Autodesk Inventor part; units mm, degrees
ref_plane "YZ Plane" through (0, 0, 0) normal (1, 0, 0) x (0, 1, 0)
ref_plane "XZ Plane" through (0, 0, 0) normal (0, 1, 0) x (-1, 0, 0)
ref_plane "XY Plane" through (0, 0, 0) normal (0, 0, 1) x (1, 0, 0)
sketch "Sketch1" plane through (0, 0, 0) normal (0, 1, 0) x (-1, 0, 0)
  line L0 (0, 0) -> (0, -125.2474)
  line L1 (0, -125.2474) -> (-3.4036, -125.2474)
  line L2 (0, 0) -> (-3.4036, 0)
  line L3 (-3.4036, 0) -> (-6.5786, -31.3753)
  line L4 (-6.5786, -31.3753) -> (-1.778, -62.7507)
  line L5 (-1.778, -62.7507) -> (-6.5786, -93.8721)
  line L6 (-6.5786, -93.8721) -> (-3.4036, -125.2474)
  dimension "d0" = 125.2474
  dimension "d1" = 3.4036
  dimension "d2" = 3.4036
  dimension "d3" = 31.3754
  dimension "d4" = 62.7507
  dimension "d5" = 31.3754
  dimension "d6" = 3.175
  dimension "d7" = 3.175
extrude "Extrusion1" add sketch "Sketch1" along normal blind 7.3025
sketch "Sketch2" plane through (0, 0, 0) normal (0, 0, 1) x (1, 0, 0)
  line L0 (0, 0) -> (0, 7.3025)
  line L1 (3.4036, 0) -> (0, 0)
  line L2 (0, 7.3025) -> (1.651, 7.3025)
  line L3 (1.651, 7.3025) -> (1.651, 0)
  line L4 (1.651, 0) -> (0, 0)
  line L5 (0, 0) -> (0, 7.3025)
  dimension "d10" = 1.651
sketch "Sketch3" plane through (3.4036, 0, -125.2474) normal (0, 0, -1) x (-1, 0, 0)
  line L0 (0, 0) -> (3.4036, 0)
  line L1 (3.4036, 7.3025) -> (1.7526, 7.3025)
  line L2 (1.7526, 7.3025) -> (1.7526, 0)
  line L3 (1.7526, 0) -> (3.4036, 0)
  line L4 (3.4036, 0) -> (3.4036, 7.3025)
  dimension "d11" = 1.651
extrude "Extrusion2" add sketch "Sketch2" along normal blind 2.5654
extrude "Extrusion3" add sketch "Sketch3" along normal blind 2.5654
properties part number "long_insert_CPY1"
Could you check a few things on this model? Use its own coordinates, in mm. A direction names the side the tool comes from. Round coordinates to 2 decimals unless told otherwise and drop trailing zeros. Loops run counter-clockwise (first coordinate to the right, second up) from the corner with the lowest first, then second, coordinate; pieces in that order, holes last. Notation, with made-up numbers: (-7, -39) - (-3, -39) arc R6 cw to (-3, -31) - close; hole circle Ø3 at (32.5, 75). An arc over 180 degrees is marked (long way). Answer in a Markdown table with one row per item. Add a question column.
(1) I'm going to push flat-ended pins straight in: pin 1 (4 mm diameter, centred on y = 2, z = -15, fed in from +X); pin 2 (0.9 mm diameter, centred on x = 2.5, y = 5, fed in from +Z); pin 3 (3 mm diameter, centred on y = 6.5, z = -37, fed in from +X). Where does each tip first touch, or does it pass through?
(2) For faces 1 (the face through (1.651, 4, -127)), 2 (the face through (0, 4, -62)), which set-ups out of +Z, -Z, +X, -X, +Y, -Y let a thin tool reach every point of the face, with its end or its side?
(3) If we section it at C-C (z = -112.5): Please give me the cut outline in (x, y).
(4) I need wall thicknesses on line 1 along X through (y, z) = (2.75, -113); line 2 along X through (y, z) = (1, -56). Which ranges of each line are inside material? Lowest first, please.
(5) If we mould it in two halves opening along Z, with no side actions, what happens to faces 3 (the face through (4.145, 3.6, -78.094)), 4 (the face through (4.212, 3.6, -46.843)), 5 (the face through (1.651, 4, 1)), 6 (the face through (5.013, 3.6, -109.34))? For each: pulls with the +Z half, pulls with the -Z half, needs draft (parallel to the pull), parting line crosses it, or undercut.
(6) If we section it at A-A (y = 4): Please give me the cut outline in (x, z), plus the area to 3 significant figures.
(7) If we section it at B-B (z = -5.5): Please give me the cut outline in (x, y).
Model answer:
| question | item | result |
|---|---|---|
| 1 | pin 1 | stops at x = 5.12 |
| 1 | pin 2 | stops at z = 0 |
| 1 | pin 3 | stops at x = 5.95 |
| 2 | face 1 | -Z, +X, +Y, -Y |
| 2 | face 2 | +Z, -Z, -X, +Y, -Y |
| 3 | outline | (0, 0) - (4.69, 0) - (4.69, 7.3) - (0, 7.3) - close |
| 4 | line 1 | x = 0 to 4.64 |
| 4 | line 2 | x = 0 to 2.81 |
| 5 | face 3 | undercut |
| 5 | face 4 | undercut |
| 5 | face 5 | needs draft |
| 5 | face 6 | pulls with the -Z half |
| 6 | outline | (0, -127.81) - (1.65, -127.81) - (1.65, -125.25) - (3.4, -125.25) - (6.58, -93.87) - (1.78, -62.75) - (6.58, -31.38) - (3.4, 0) - (1.65, 0) - (1.65, 2.57) - (0, 2.57) - close |
| 6 | area | 583 mm² |
| 7 | outline | (0, 0) - (3.96, 0) - (3.96, 7.3) - (0, 7.3) - close |
